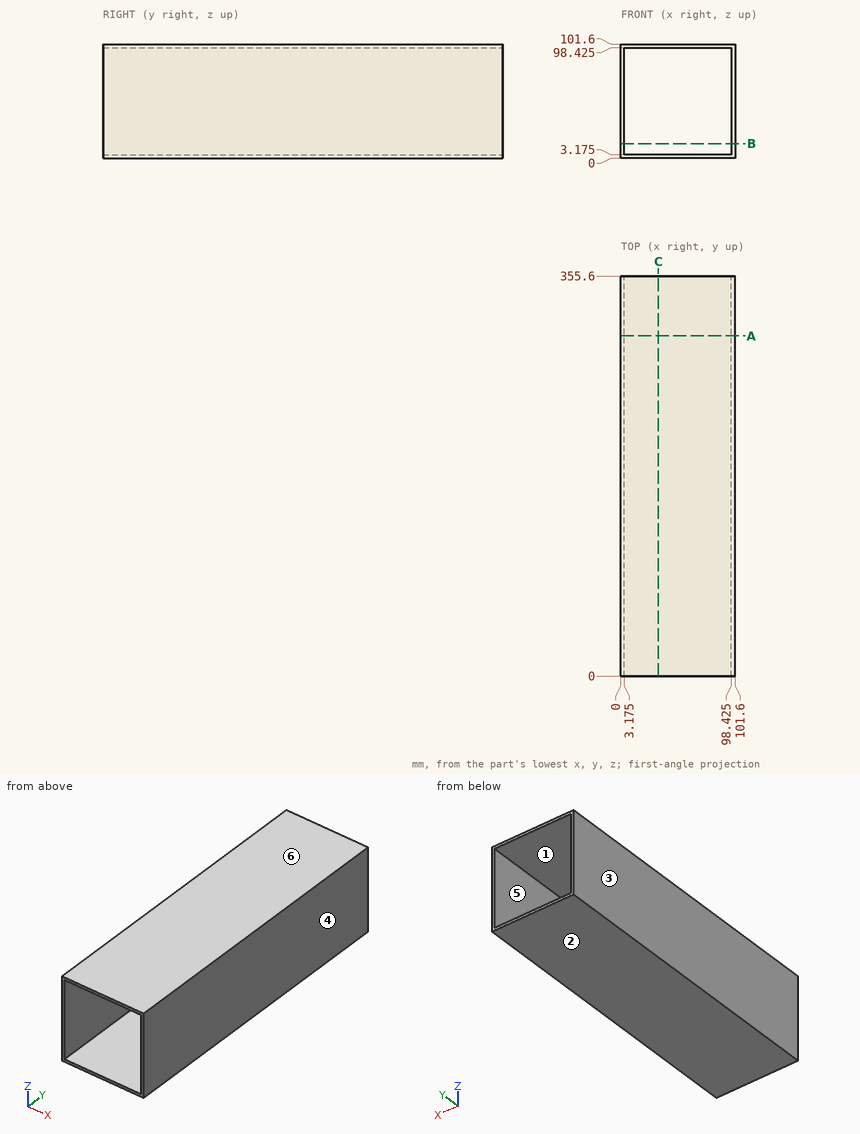
Here's the drawing with two shaded views (mm, measured from the low corner). I have some questions. A direction names the side the tool comes from. Coordinates: 2 decimals unless noted, no trailing zeros. Order: outer loops, then holes, each group sorted by start corner. A loop starts at its lowest first (then second) coordinate and runs counter-clockwise, first axis right, second up.
Q1. Suppose I cut it at B-B on z = 13. Please give me the cut outline in (x, y) (3 decimals).
Q2. Suppose I cut it at A-A on y = 302.5. Please give me the cut outline in (x, z) (3 decimals), and give its area (3 significant figures).
Q3. Please list where this line runs through material, in increasing order: L1, parallel to X at y = 322, z = 73 (3 decimals).
Q4. Suppose I cut it at C-C on x = 33.5. Please give me the cut outline in (y, z) (3 decimals).
Q5. Which directions (+Z, -Z, +X, -X, +Y, -Y) give clear straight access to the entire face, cutting with the end or side of a thin tool? Please do the marked faces 5 and 6.
Q6. Thinking about a two-plate mould opening in X: for the marked faces 1, 2, 3 and 4, which applies, released by +X, released by -X, zero draft, split by the parting line, or undercut?
Answer:
1. outline: (0, 0) - (3.175, 0) - (3.175, 355.6) - (0, 355.6) - close; (98.425, 0) - (101.6, 0) - (101.6, 355.6) - (98.425, 355.6) - close
2. outline: (0, 0) - (101.6, 0) - (101.6, 101.6) - (0, 101.6) - close; hole (3.175, 3.175) - (98.425, 3.175) - (98.425, 98.425) - (3.175, 98.425) - close
2. area: 1,250 mm2
3. L1: x = 0 to 3.175, 98.425 to 101.6
4. outline: (0, 0) - (355.6, 0) - (355.6, 3.175) - (0, 3.175) - close; (0, 98.425) - (355.6, 98.425) - (355.6, 101.6) - (0, 101.6) - close
5. face 5: +Y, -Y
5. face 6: +Z, +X, -X, +Y, -Y
6. face 1: undercut
6. face 2: zero draft
6. face 3: released by -X
6. face 4: released by +X
